from build123d import *

# Parameters (mm, degrees)
F1_DEPTH = 150
F2_DEPTH = 25
F2_TAPER = -20


with BuildPart() as f1:
    # F0 (on Front) → F1 (new body)
    with BuildSketch(Plane.XZ):
        Polygon((-0.4338717465, 24.399797494), (-13.9581263065, 13.9433988455), (-8.1927247302, -2.1501364642), (-3.8462013472, -2.020396331), (3.8462013472, -1.7907844638), (8.8947439628, -1.6400896363), (13.6899788204, 14.7686719489), align=None)
        Polygon((3.8462013472, -1.7907844638), (-3.8462013472, -2.020396331), (-3.8462013472, -4.5691458424), (-1.3902849751, -4.5691458424), (-1.3902849751, -9.7131561403), (0, -9.7131561403), (1.3902849751, -9.7131561403), (1.3902849751, -4.5691458424), (3.8462013472, -4.5691458424), align=None)
    extrude(amount=F1_DEPTH)

    # F1_face (on face) → F2 (join)
    with BuildSketch(Plane(origin=(0.0021061426, -150, 8.9125586463), x_dir=(1, 0, 0), z_dir=(0, -1, 0))):
        Polygon((-8.1948308728, -11.0626951105), (-3.8483074898, -10.9329549773), (-3.8483074898, -13.4817044887), (-1.3923911176, -13.4817044887), (-1.3923911176, -18.6257147866), (1.3881788325, -18.6257147866), (1.3881788325, -13.4817044887), (3.8440952046, -13.4817044887), (3.8440952046, -10.7033431101), (8.8926378202, -10.5526482826), (13.6878726779, 5.8561133027), (-0.4359778891, 15.4872388477), (-13.9602324491, 5.0308401992), align=None)
    extrude(amount=F2_DEPTH, taper=F2_TAPER)


solid = f1.part
Part model, mm, in its own coordinate system. A direction names the side the tool comes from. Round coordinates to 2 decimals unless told otherwise and drop trailing zeros. Write each loop counter-clockwise with the first axis right and the second up, starting at its lowest first coordinate (ties: lowest second). Pieces come first, ordered by that corner, then holes. Notation, with made-up numbers: M 74,57 L 111,57 A18 ccw 111,70 Z; hole C 5.5,-25 d11. An arc over 180 degrees is marked long. Return JSON: item names as keys, results as strings. Group by question number.
(1) Drill centre lines: probe 1 along X at (y, z) = (-43, -9.5); probe 2 along Z at (x, y) = (-3.5, -138); probe 3 along X at (y, z) = (-103.5, 17.5). Where is each one in solid material? Low to high.
(2) Pin check, flat tips, straight feed: pin 1 Ø8 at (x, y) = (10.5, -86) entering from +Z; pin 2 Ø2 at (y, z) = (-58, -3) entering from +X; pin 3 Ø10 at (x, y) = (12, -152) entering from +Z. Stop position of each tip, or through.
(3) Which spindle directions (+Z, -Z, +X, -X, +Y, -Y) get a long thin tool onto all of the face, cutting with end or side? Do faces 1 (the face through (-1.39, -74, -7)), 2 (the face through (6.727, -73.95, 19.517)), 3 (the face through (-7.101, -73.95, 19.245)), 4 (the face through (11.26, -73.95, 6.45)), 5 (the face through (2, -175, 6)). Say none if no direction does.
(4) Saw through at A-A on y = -103. Write the cut outline in (x, z), then the cut area to 3 significant figures.
Returned:
{
 "1": {"probe 1": "-1.39 to 1.39", "probe 2": "-4.57 to 22.03", "probe 3": "-9.36 to 9.68"},
 "2": {"pin 1": "z = 19.67", "pin 2": "x = 3.85", "pin 3": "z = 20.86"},
 "3": {"face 1": "-Z, -X, +Y", "face 2": "+Z, +X, +Y", "face 3": "+Z, -X, +Y", "face 4": "-Z, +X, +Y", "face 5": "+Z, -Z, +X, -X, -Y"},
 "4": {"outline": "M -13.96,13.94 L -8.19,-2.15 L -3.85,-2.02 L -3.85,-4.57 L -1.39,-4.57 L -1.39,-9.71 L 1.39,-9.71 L 1.39,-4.57 L 3.85,-4.57 L 3.85,-1.79 L 8.89,-1.64 L 13.69,14.77 L -0.43,24.4 Z", "area": "538 mm²"}
}
